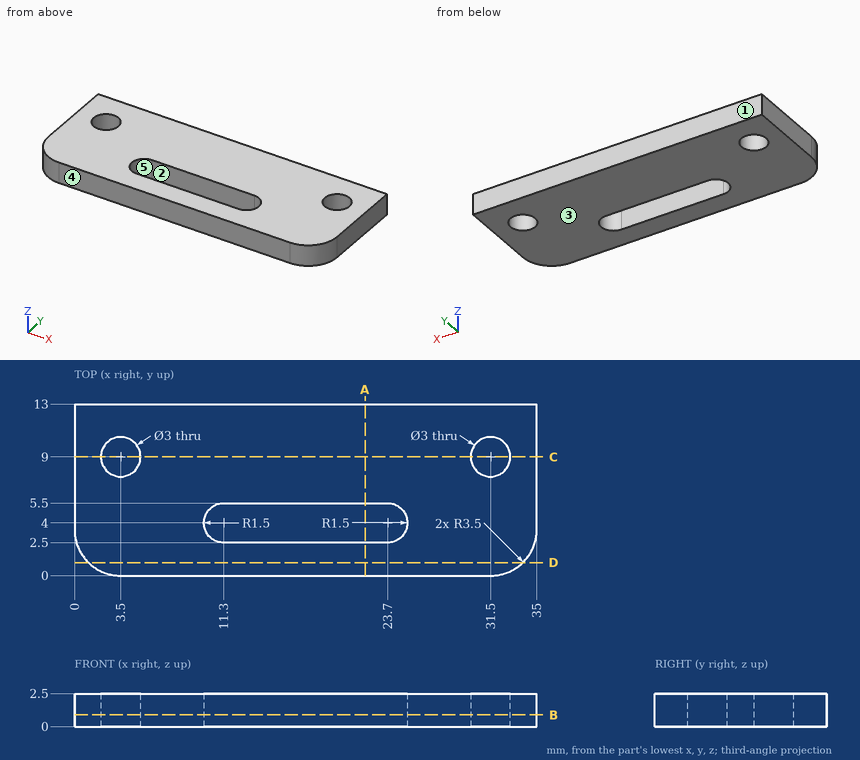
Geometry: see drawing. Coordinates: mm, zero at the bounding-box minimum. A direction names the side the tool comes from. Round coordinates to 2 decimals unless told otherwise and drop trailing zeros. Write each loop counter-clockwise with the first axis right and the second up, starting at its lowest first coordinate (ties: lowest second). Pieces come first, ordered by that corner, then holes.
1) Cut plane C-C (y = 9). Return the cut outline in (x, z), then the cut area to 3 significant figures.
2) Cut plane A-A (x = 22). Return the cut outline in (y, z), then the cut area to 3 significant figures.
3) Cut plane D-D (y = 1). Return the cut outline in (x, z).
4) Cut plane B-B (z = 0.9). Return the cut outline in (x, y).
5) Reachability of the marked faces 1 and 2 from +Z, -Z, +X, -X, +Y, -Y: full face, straight path, thin tool, end or side. Return the list, or none.
6) Draft query along Y for the marked faces 3, 4 and 5. Return one class per face: pulls with the +Y half, pulls with the -Y half, needs draft (parallel to the pull), parting line crosses it, or undercut.
7) Contact query for flat-ended pins moving along their axis: P1, Ø1, axis at x = 17, y = 8.5, coming from the -Z side; P2, Ø2.5, axis at x = 31.5, y = 9, coming from the -Z side. Output: stop coordinate, or through.
8) Ray query, L1, parallel to Y at x = 31.5, z = 1.2; L2, parallel to X at y = 8.5, z = 0.7; L3, parallel to Y at x = 19.5, z = 1.8. Return the intervals inside material, ascending.
Geometry says:
1. outline: (0, 0) - (2, 0) - (2, 2.5) - (0, 2.5) - close; (5, 0) - (30, 0) - (30, 2.5) - (5, 2.5) - close; (33, 0) - (35, 0) - (35, 2.5) - (33, 2.5) - close
1. area: 72.5 mm2
2. outline: (0, 0) - (2.5, 0) - (2.5, 2.5) - (0, 2.5) - close; (5.5, 0) - (13, 0) - (13, 2.5) - (5.5, 2.5) - close
2. area: 25.0 mm2
3. outline: (1.05, 0) - (33.95, 0) - (33.95, 2.5) - (1.05, 2.5) - close
4. outline: (0, 3.5) arc R3.5 ccw to (3.5, 0) - (31.5, 0) arc R3.5 ccw to (35, 3.5) - (35, 13) - (0, 13) - close; hole circle Ø3 at (3.5, 9); hole (11.3, 2.5) - (23.7, 2.5) arc R1.5 ccw to (23.7, 5.5) - (11.3, 5.5) arc R1.5 ccw to start; hole circle Ø3 at (31.5, 9)
5. face 1: +Z, -Z, +X, -X, +Y
5. face 2: +Z, -Z
6. face 3: needs draft
6. face 4: pulls with the -Y half
6. face 5: undercut
7. P1: stops at z = 0
7. P2: passes through
8. L1: y = 0 to 7.5, 10.5 to 13
8. L2: x = 0 to 2.09, 4.91 to 30.09, 32.91 to 35
8. L3: y = 0 to 2.5, 5.5 to 13
